Input: part model. Units: mm. Frame: model coordinates. Face numbers are marked on the shaded views. A direction names the side the tool comes from. Coordinates: 2 decimals unless noted, no trailing zeros. Write each loop counter-clockwise with the first axis right and the second up, starting at its lowest first coordinate (ties: lowest second). Pieces come first, ordered by that corner, then holes.
1) Section query C-C (y = 24). Output: boundary loops of the cut face in (x, z).
2) Section query B-B (z = -15). Output: boundary loops of the cut face in (x, y) (3 decimals).
3) Pin query (flat end, axial travel): pin 1 Ø4 at (x, y) = (-9, 38.5) entering from +Z; pin 2 Ø2.5 at (x, y) = (-8.6, 39.125) entering from -Z; pin 3 Ø3 at (x, y) = (-8.5, 39.5) entering from -Z. Return the tip coordinate at first contact, or that it passes through.
4) Set-up query: the marked faces 4, 5 and 6. Return all of +Z, -Z, +X, -X, +Y, -Y with unobstructed straight access to the full face (end or side cutting, diameter ignored); none if empty.
5) Draft query along Y for the marked faces 1, 2 and 3. Return one class per face: pulls with the +Y half, pulls with the -Y half, needs draft (parallel to the pull), parting line crosses it, or undercut.
6) Line query: L1, parallel to Y at x = -8.6, z = -12.6 (3 decimals); L2, parallel to Y at x = 4, z = -5.5; L3, parallel to X at y = 9.5, z = -23. Output: solid intervals per line, ascending.
7) Section query A-A (x = -6.5). Output: boundary loops of the cut face in (y, z), then the cut area to 3 significant figures.
8) Section query D-D (z = -23). Output: boundary loops of the cut face in (x, y).
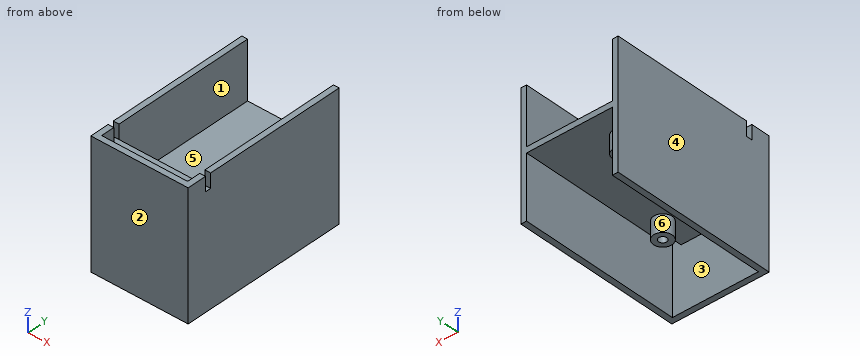
Autodesk Inventor part; units mm, degrees
ref_plane "bottom of connector plate" through (0, -2, 0) normal (0, 1, 0) x (-1, 0, 0)
ref_plane "YZ Plane" through (0, 0, 0) normal (1, 0, 0) x (0, 1, 0)
ref_plane "XY Plane" through (0, 0, 0) normal (0, 0, 1) x (1, 0, 0)
ref_plane "bottom of connector plate" through (0, -2, 0) normal (0, 1, 0) x (-1, 0, 0)
sketch "Sketch1" plane through (0, 0, 0) normal (0, 1, 0) x (-1, 0, 0)
  line L0 (17, -11) -> (-17, -11)
  line L1 (-17, -11) -> (-17, 11)
  line L2 (-17, 11) -> (17, 11)
  line L3 (17, 11) -> (17, -11)
  line L4 (17, -11) -> (-17, 11) construction
  line L5 (-17, -11) -> (17, 11) construction
  line L6 (15, -9) -> (-15, -9)
  line L7 (-15, -9) -> (-15, 9)
  line L8 (-15, 9) -> (15, 9)
  line L9 (15, 9) -> (15, -9)
  line L10 (15, -9) -> (-15, 9) construction
  line L11 (-15, -9) -> (15, 9) construction
  line L12 (17, -11) -> (-17, -11)
  line L13 (-17, -11) -> (-17, -33)
  line L14 (-17, -33) -> (17, -33)
  line L15 (17, -33) -> (17, -11)
  line L16 (15, -11) -> (-15, -11)
  line L17 (-15, -11) -> (-15, -26)
  line L18 (-15, -26) -> (15, -26)
  line L19 (15, -26) -> (15, -11)
  line L20 (15, 9) -> (15, 11)
  line L21 (-15, 9) -> (-15, 11)
  line L22 (-15, -26) -> (-15, -33)
  line L23 (15, -26) -> (15, -33)
  line L24 (15, -9) -> (17, -9)
  line L25 (-15, -9) -> (-17, -9)
  point P0 (0, 0)
  dimension "d0" = 34
  dimension "d1" = 22
  dimension "d2" = 30
  dimension "d3" = 18
  dimension "d5" = 22
  dimension "d6" = 15
extrude "top" add sketch "Sketch1" along normal blind 50 contours L15 L14 L23 L19 L0 | L0 L1 L25 L6 L24 L3 | L24 L9 L20 L2 L3 | L17 L22 L14 L13 L0 | L25 L1 L2 L21 L7
sketch "Sketch2" plane through (0, 0, 0) normal (0, 1, 0) x (-1, 0, 0)
  line L0 (17, -33) -> (17, 6)
  line L1 (-17, 11) -> (-17, -33)
  line L2 (17, 6) -> (-17, 6)
  line L3 (-17, 6) -> (-17, -33)
  line L4 (-17, -28) -> (17, -28)
  line L5 (17, -28) -> (17, 11)
  line L6 (-15, -11) -> (15, -11)
  line L7 (15, -26) -> (-15, -26)
  line L8 (15, -11) -> (-15, -11)
  line L9 (-15, -11) -> (-15, -26)
  line L10 (-15, -26) -> (15, -26)
  line L11 (15, -26) -> (15, -11)
  line L12 (15, 11) -> (15, -9)
  line L13 (-15, -9) -> (-15, 11)
  line L14 (15, -9) -> (-15, -9)
  line L15 (-15, -9) -> (-15, 11)
  line L16 (-15, 11) -> (15, 11)
  line L17 (15, 11) -> (15, -9)
  circle A0 centre (6.5, 0) radius 4.8
  circle A1 centre (-6.5, 0.1042) radius 4.8
  line L18 (6.5, 0) -> (0, 0) construction
  line L19 (-15, -26) -> (-15, -28)
  line L20 (15, -26) -> (15, -28)
  line L21 (-17, -33) -> (17, -33)
  line L22 (-15, -28) -> (-15, -33)
  line L23 (15, -28) -> (15, -33)
  point P0 (17, -9)
  point P1 (-17, -9)
  point P2 (17, 6)
  dimension "d10" = 9.6
  dimension "d11" = 9.6
  dimension "d12" = 13
  dimension "d13" = 6.5
extrude "plate" add sketch "Sketch2" against normal blind 2 contours L21 L23 L4 L0 | L4 L20 L11 L6 L9 L19 L1 L2 L13 L14 L12 L0 | L21 L1 L4 L22 | L12 L14 L13 L2
sketch "Sketch3" plane through (0, -2, 0) normal (0, 1, 0) x (-1, 0, 0)
  line L0 (17, 11) -> (17, -28)
  line L1 (17, -28) -> (-17, -28)
  line L2 (17, 11) -> (-17, 11)
  line L3 (-17, 11) -> (-17, -28)
  line L4 (-17, -28) -> (17, -28)
  line L5 (17, -28) -> (17, 11)
  line L6 (-15, -26) -> (15, -26)
  line L7 (15, 11) -> (15, -9)
  line L8 (-15, -26) -> (15, -26)
  line L9 (15, -26) -> (15, 9)
  line L10 (15, 9) -> (-15, 9)
  line L11 (-15, 9) -> (-15, -26)
  line L12 (15, 11) -> (15, -9)
  line L13 (15, 9) -> (15, 11)
  line L14 (-15, -9) -> (-15, 11)
  line L15 (-15, 9) -> (-15, 11)
  line L16 (-15, -11) -> (15, -11)
  line L17 (17, -9) -> (-17, -9)
  line L18 (15, -11) -> (-15, -11)
  line L19 (-15, -11) -> (-15, -9)
  line L20 (-15, -9) -> (15, -9)
  line L21 (15, -9) -> (15, -11)
  line L22 (-15, -26) -> (-15, -28)
  line L23 (15, -26) -> (15, -28)
  line L24 (-17, -28) -> (-17, -33)
  line L25 (-17, -33) -> (-15, -33)
  line L26 (-15, -33) -> (-15, -28)
  line L27 (17, -28) -> (17, -33)
  line L28 (17, -33) -> (15, -33)
  line L29 (15, -33) -> (15, -28)
  line L30 (-15, -33) -> (15, -33)
  point P0 (0, 0)
  point P1 (15, -26)
  dimension "d17" = 35
  dimension "d45" = 5
  dimension "d46" = 2
  dimension "d47" = 5
  dimension "d48" = 2
extrude "base" add sketch "Sketch3" against normal blind 4.75 contours L0 L17 L7 L2 | L0 L1 L23 L9 L17 | L27 L28 L29 L1 | L9 L16 L11 L17 | L14 L11 L17 L3 L2 | L11 L22 L1 L3 L17 | L26 L25 L24 L1
sketch "Sketch6" plane through (-15, -8.75, -9) normal (0, 0, 1) x (1, 0, 0)
  line L0 (30, 2) -> (30, 58.75)
  line L1 (30, 2) -> (27, 2)
  line L2 (27, 2) -> (27, 5)
  line L3 (27, 5) -> (30, 5)
  line L4 (30, 5) -> (30, 2)
  line L5 (16.5, 5) -> (16.5, 2)
  line L6 (13.5, 5) -> (13.5, 2)
  line L7 (13.5, 5) -> (16.5, 5)
  line L8 (16.5, 2) -> (13.5, 2)
  point P0 (15, 8.75)
  dimension "d23" = 3
  dimension "d24" = 3
extrude "Extrusion4" cut sketch "Sketch6" against normal blind 2
sketch "Sketch5" plane through (0, -6.75, 0) normal (0, 1, 0) x (-1, 0, 0)
  line L0 (17, 11) -> (-17, 11)
  line L1 (-17, 11) -> (-17, -28)
  line L2 (-17, -28) -> (17, -28)
  line L3 (17, -28) -> (17, 11)
  line L4 (-17, -28) -> (-17, -33)
  line L5 (-17, -33) -> (17, -33)
  line L6 (17, -33) -> (17, -28)
  dimension "d49" = 39
  dimension "d50" = 5
extrude "Extrusion5" add sketch "Sketch5" against normal blind 2
ref_plane "Work Plane4" through (0, -32.5, 0) normal (0, 1, 0) x (-1, 0, 0)
sketch "Sketch4" plane through (0, -32.5, 0) normal (0, 1, 0) x (-1, 0, 0)
  line L0 (-15, 11) -> (15, 11)
  line L1 (-17, -33) -> (17, -33)
  line L2 (17, 11) -> (-17, -33) construction
  circle A0 centre (0, -8.5) radius 12
  point P0 (0, 0)
  dimension "d22" = 24
sketch "Sketch7" plane through (15, 50, -11) normal (0, 0, -1) x (-1, 0, 0)
  line L0 (30, -56.75) -> (0, -56.75)
  line L1 (3, -3.375) -> (27, -3.375) construction
  line L2 (27, -3.375) -> (27, -53.375) construction
  line L3 (27, -53.375) -> (3, -53.375) construction
  line L4 (3, -53.375) -> (3, -3.375) construction
  line L5 (3, -3.375) -> (27, -53.375) construction
  line L6 (27, -3.375) -> (3, -53.375) construction
  circle A0 centre (-12.1992, -48.387) radius 1.4
  circle A1 centre (-12.1992, -48.387) radius 3.25
  circle A2 centre (6.4, -45.875) radius 1.4
  circle A3 centre (6.4, -45.875) radius 3.25
  circle A4 centre (23.6, -10.875) radius 1.4
  circle A5 centre (23.6, -10.875) radius 3.25
  point P0 (15, -50)
  point P1 (15, -28.375)
  dimension "d31" = 24
  dimension "d32" = 50
  dimension "d33" = 2.8
  dimension "d34" = 6.5
  dimension "d35" = 2.8
  dimension "d36" = 6.5
  dimension "d37" = 2.8
  dimension "d38" = 6.5
  dimension "d39" = 7.5
  dimension "d40" = 3.4
  dimension "d41" = 7.5
  dimension "d42" = 3.4
extrude "Extrusion6" add sketch "Sketch7" along normal blind 6 contours A3 | A5
properties part number "Tclamp_enclosure_3DPrint"
Answer:
1. outline: (-17, -33) - (-15, -33) - (-15, -11) - (15, -11) - (15, -33) - (17, -33) - (17, 11) - (15, 11) - (15, -9) - (-15, -9) - (-15, 11) - (-17, 11) - close
2. outline: (-17, -8.75) - (17, -8.75) - (17, 50) - (15, 50) - (15, -6.75) - (-15, -6.75) - (-15, 50) - (-17, 50) - close; circle Ø6.5 at (-8.6, 39.125); circle Ø6.5 at (8.6, 4.125); hole circle Ø2.8 at (-8.6, 39.125); hole circle Ø2.8 at (8.6, 4.125)
3. pin 1: stops at z = -9
3. pin 2: stops at z = -11
3. pin 3: stops at z = -17
4. face 4: +Z, -Z, -X, +Y, -Y
4. face 5: +Z, +Y
4. face 6: -Z
5. face 1: needs draft
5. face 2: pulls with the -Y half
5. face 3: undercut
6. L1: y = -8.75 to -6.75, 35.875 to 37.725, 40.525 to 42.375
6. L2: y = -8.75 to -6.75, -2 to 0
6. L3: x = -17 to -15, 15 to 17
7. outline: (-8.75, -33) - (-6.75, -33) - (-6.75, -11) - (36.64, -11) - (36.64, -17) - (41.61, -17) - (41.61, -11) - (50, -11) - (50, -9) - (0, -9) - (0, -4.8) - (-2, -4.8) - (-2, -9) - (-6.75, -9) - (-6.75, 11) - (-8.75, 11) - close; (-2, 4.8) - (0, 4.8) - (0, 6) - (-2, 6) - close
7. area: 242 mm2
8. outline: (-17, -8.75) - (17, -8.75) - (17, 50) - (15, 50) - (15, -6.75) - (-15, -6.75) - (-15, 50) - (-17, 50) - close
